from build123d import *

# Parameters (mm, degrees)
ESBO_O1_R                = 20
ESBO_O1_R_2              = 4
RESSALTO_EXTRUS_O3_DEPTH = 3
ESBO_O1_6_R              = 22
ESBO_O1_6_R_2            = 20
RESSALTO_EXTRUS_O4_DEPTH = 6
ESBO_O1_7_R              = 4
RESSALTO_EXTRUS_O5_DEPTH = 2


with BuildPart() as part:
    # Esboço1 → Ressalto-extrusão3 (new body)
    with BuildSketch(Plane.XY):
        Circle(ESBO_O1_R)
        Circle(ESBO_O1_R_2, mode=Mode.SUBTRACT)
    extrude(amount=RESSALTO_EXTRUS_O3_DEPTH)

    # Esboço1<6> → Ressalto-extrusão4 (add)
    with BuildSketch(Plane.XY):
        Circle(ESBO_O1_6_R)
        Circle(ESBO_O1_6_R_2, mode=Mode.SUBTRACT)
    extrude(amount=RESSALTO_EXTRUS_O4_DEPTH)

    # Esboço1<7> → Ressalto-extrusão5 (add)
    with BuildSketch(Plane.XY):
        Circle(ESBO_O1_7_R)
    extrude(amount=RESSALTO_EXTRUS_O5_DEPTH)


solid = part.part
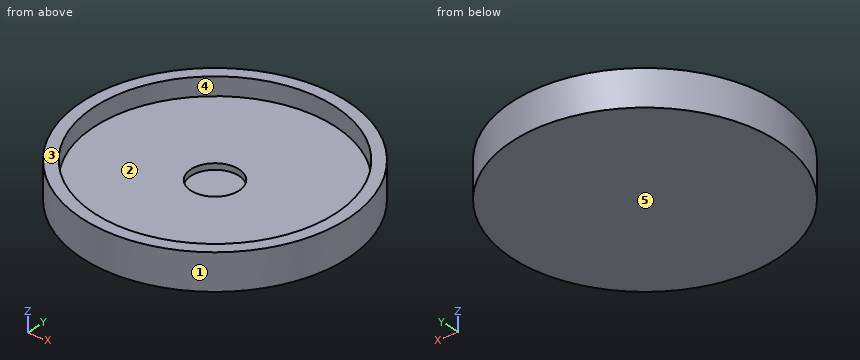
Here's how the part is built. I have some questions about the finished solid (model axes, mm). Face numbers are marked on the shaded views. A direction names the side the tool comes from. Give positions to 0.01 mm unless a question says otherwise; leave off trailing zeros. Loops run counter-clockwise (first coordinate to the right, second up) from the corner with the lowest first, then second, coordinate; pieces in that order, holes last. Notation, with made-up numbers: (66.25, 79.25) -> (104.25, 79.25) arc R18 ccw to (104.25, 105.25) -> close; hole circle Ø10 at (42.25, -8). An arc over 180 degrees is marked (long way). One line per item, written item: value.
Q1. Suppose I cut it at D-D on z = 4.65. Please give me the cut outline in (x, y), then the cut area to 3 significant figures.
Answers follow:
outline: circle Ø44 at (0, 0); hole circle Ø40 at (0, 0)
area: 264 mm^2
Q2. I'm going to push flat-ended pins straight in: pin 1 Ø2 at (x, y) = (-8.5, 11) entering from +Z; pin 2 Ø7 at (x, y) = (0, 0) entering from -Z. Where does each tip first touch, or does it pass through?
Answers follow:
pin 1: z = 3
pin 2: z = 0
Q3. If I drill on line 1 along Y through (x, z) = (0, 2.45); line 2 along Z through (x, y) = (-8.5, 10); line 3 along Y through (x, z) = (0, 4.45), over which ranges is the centre line in solid material (lowest first)?
Answers follow:
line 1: -22 to -4, 4 to 22
line 2: 0 to 3
line 3: -22 to -20, 20 to 22
Q4. On a 3-axis mill with a long thin cutter (end or side, diameter ignored), from which of +Z, -Z, +X, -X, +Y, -Y can I reach the whole of each face in a straight line? I mean the marked faces 4 and 5. Say none if no direction works.
Answers follow:
face 4: +Z
face 5: -Z, +X, -X, +Y, -Y
Q5. Suppose I cut it at C-C on z = 1.35. Please give me the cut outline in (x, y).
Answers follow:
outline: circle Ø44 at (0, 0)
Q6. Suppose I cut it at A-A on x = 0. Please give me the cut outline in (y, z), then the cut area to 3 significant figures.
Answers follow:
outline: (-22, 0) -> (22, 0) -> (22, 6) -> (20, 6) -> (20, 3) -> (4, 3) -> (4, 2) -> (-4, 2) -> (-4, 3) -> (-20, 3) -> (-20, 6) -> (-22, 6) -> close
area: 136 mm^2
Q7. We'd pull the mould along X, two halves only. Please class the marked faces 1, 2 and 3: pulls with the +X half, pulls with the -X half, needs draft (parallel to the pull), parting line crosses it, or undercut.
Answers follow:
face 1: parting line crosses it
face 2: undercut
face 3: needs draft
